Autodesk Fusion 360 part; units mm, degrees
sketch "Sketch1" plane through (0, 0, 0) normal (0, 0, 1) x (1, 0, 0)
  arc A0 (0.1047, -30.3528) -> (-0.0415, 30.353) centre (0, 0) ccw
  line L0 (-0.0415, 30.353) -> (-0.0415, 62.103)
  line L1 (0.1047, -30.3528) -> (0.1047, -62.1028)
  line L2 (-0.0415, 62.103) -> (57.1085, 62.103)
  line L3 (0.1047, -62.1028) -> (57.2547, -62.1028)
  line L4 (57.1085, 62.103) -> (57.2547, -62.1028)
  dimension "d1" = 60.706
  dimension "d10" = 31.75
  dimension "d12" = 57.15
extrude "Extrude1" add sketch "Sketch1" along normal mid plane 127
sketch "Sketch4" plane through (57.1815, 0.0673, 0) normal (1, 0.0012, 0) x (-0.0012, 1, 0)
  line L0 (62.0357, -63.5) -> (62.0357, 63.5)
  line L1 (62.0357, 63.5) -> (-62.1702, 63.5)
  line L2 (-62.1702, 63.5) -> (-62.1702, -63.5)
  line L3 (-62.1702, -63.5) -> (62.0357, -63.5)
  line L4 (57.15, -57.15) -> (-57.15, -57.15)
  line L5 (-57.15, -57.15) -> (-57.15, 57.15)
  line L6 (-57.15, 57.15) -> (-2.54, 57.15)
  line L7 (57.15, 6.35) -> (57.15, -57.15)
  line L8 (57.15, -57.15) -> (-57.15, 57.15) construction
  line L9 (-57.15, -57.15) -> (57.15, 57.15) construction
  line L10 (-2.54, 57.15) -> (-2.54, 6.35)
  line L11 (-2.54, 6.35) -> (57.15, 6.35)
  dimension "d21" = 114.3
  dimension "d22" = 114.3
  dimension "d35" = 59.69
  dimension "d36" = 50.8
extrude "Extrude3" cut sketch "Sketch4" against normal blind 25.4 contours L4 L5 L6 L7 L10 L11
sketch "Sketch6" plane through (57.1815, 0.0673, 0) normal (1, 0.0012, 0) x (-0.0012, 1, 0)
  line L0 (-57.15, 57.15) -> (-2.54, 57.15)
  line L1 (-2.54, 57.15) -> (-2.54, 6.35)
  line L2 (-2.54, 6.35) -> (57.15, 6.35)
  line L3 (57.15, 6.35) -> (57.15, -57.15)
  line L4 (57.15, -57.15) -> (-57.15, -57.15)
  line L5 (-57.15, -57.15) -> (-57.15, 57.15)
  line L6 (62.0357, -63.5) -> (62.0357, 63.5)
  line L7 (62.0357, 63.5) -> (-62.1702, 63.5)
  line L8 (-62.1702, 63.5) -> (-62.1702, -63.5)
  line L9 (-62.1702, -63.5) -> (62.0357, -63.5)
  line L10 (1.27, 57.15) -> (57.15, 57.15)
  line L11 (57.15, 57.15) -> (57.15, 8.89)
  line L12 (57.15, 8.89) -> (1.27, 8.89)
  line L13 (1.27, 8.89) -> (1.27, 57.15)
  dimension "d37" = 55.88
  dimension "d38" = 48.26
extrude "Extrude5" cut sketch "Sketch6" against normal blind 25.4 contours L10 L11 L12 L13
sketch "Sketch8" plane through (0, 0, 63.5) normal (0, 0, 1) x (-1, 0, 0)
  line L0 (-0.1047, 30.3528) -> (-0.1047, 62.1028)
  line L1 (-0.1047, 62.1028) -> (-57.2547, 62.1028)
  line L2 (-57.2547, 62.1028) -> (-57.1085, -62.103)
  line L3 (-57.1085, -62.103) -> (0.0415, -62.103)
  line L4 (0.0415, -62.103) -> (0.0415, -30.353)
  arc A0 (-0.1047, 30.3528) -> (0.0415, -30.353) centre (0, 0) ccw
  circle A1 centre (-49.9987, -11.1079) radius 0.8001
  circle A2 centre (-49.9987, -15.6799) radius 0.8001
  line L5 (-57.18, -1.3373) -> (-31.7801, -1.3074)
  dimension "d45" = 1.6002
  dimension "d46" = 4.572
  dimension "d47" = 9.779
extrude "Extrude6" cut sketch "Sketch8" against normal up to surface (6.35 mm away) contours A1 | A2
sketch "Sketch9" plane through (0.003, -2.54, 0) normal (0.0012, -1, 0) x (1, 0.0012, 0)
  line L0 (57.1816, 6.35) -> (57.1816, 57.15)
  line L1 (57.1816, 57.15) -> (31.7816, 57.15)
  line L2 (31.7816, 57.15) -> (31.7816, 6.35)
  line L3 (31.7816, 6.35) -> (57.1816, 6.35)
  line L4 (50.8316, 44.45) -> (38.1316, 44.45)
  line L5 (38.1316, 44.45) -> (38.1316, 19.05)
  line L6 (38.1316, 19.05) -> (50.8316, 19.05)
  line L7 (50.8316, 19.05) -> (50.8316, 44.45)
  dimension "d50" = 12.7
  dimension "d51" = 25.4
  dimension "d52" = 12.7
  dimension "d54" = 6.35
extrude "Extrude7" cut sketch "Sketch9" against normal up to surface (3.81 mm away) contours L4 L5 L6 L7
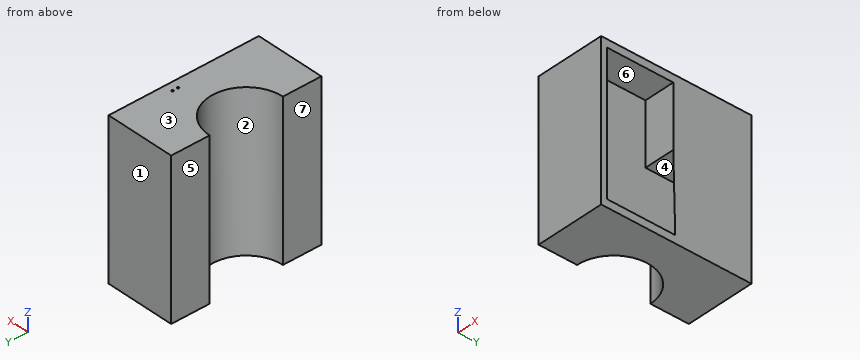
Part model, mm, in its own coordinate system. Face numbers are marked on the shaded views. A direction names the side the tool comes from. Coordinates: 2 decimals unless noted, no trailing zeros. Order: outer loops, then holes, each group sorted by start corner. A loop starts at its lowest first (then second) coordinate and runs counter-clockwise, first axis right, second up.
(1) Pull direction Y, two halves, no side cores. Call the marked faces 1, 2, 3 and 4: pulls with the +Y half, pulls with the -Y half, needs draft (parallel to the pull), parting line crosses it, or undercut.
Check sheet entries:
face 1: pulls with the +Y half
face 2: undercut
face 3: needs draft
face 4: undercut
(2) Slice it at D-D, the plane z = -5.5. Write the cut outline in (x, y), and give its area (3 significant figures).
Check sheet entries:
outline: (-0.04, 30.35) arc R30.35 cw to (0.1, -30.35) - (0.1, -62.1) - (57.25, -62.1) - (57.25, -57.08) - (31.85, -57.11) - (31.71, 57.19) - (57.11, 57.22) - (57.18, -0.84) - (57.11, 62.1) - (-0.04, 62.1) - close
area: 2,750 mm2
(3) Slice it at A-A, the plane x = 28.5. Write the cut outline in (y, z), and give its area (3 significant figures).
Check sheet entries:
outline: (-62.1, -63.5) - (-10.44, -63.5) - (-10.44, 63.5) - (-62.1, 63.5) - close; (10.44, -63.5) - (62.1, -63.5) - (62.1, 63.5) - (10.44, 63.5) - close
area: 13,100 mm2
(4) Slice it at C-C, the plane x = 41. Write the cut outline in (y, z).
Check sheet entries:
outline: (-62.1, -63.5) - (62.1, -63.5) - (62.1, 63.5) - (-62.1, 63.5) - close; hole (-57.1, -57.15) - (57.2, -57.15) - (57.2, 6.35) - (-2.49, 6.35) - (-2.49, 57.15) - (-57.1, 57.15) - close; hole (-2.49, 19.05) - (1.32, 19.05) - (1.32, 8.89) - (57.2, 8.89) - (57.2, 57.15) - (1.32, 57.15) - (1.32, 44.45) - (-2.49, 44.45) - close
(5) Probe L1, parallel to Y at x = 54.5, z = 55.5; L2, parallel to Z at x = 53.5, y = 39; L3, parallel to Z at x = 43.5, y = -3. List the from-to ranges inside material, lowest first.
Check sheet entries:
L1: y = -62.1 to -57.09, -2.48 to 1.33, 57.21 to 62.1
L2: z = -63.5 to -57.15, 6.35 to 8.89, 57.15 to 63.5
L3: z = -63.5 to -57.15, 57.15 to 63.5
(6) Slice it at B-B, the plane z = 54.5. Write the cut outline in (x, y).
Check sheet entries:
outline: (-0.04, 30.35) arc R30.35 cw to (0.1, -30.35) - (0.1, -62.1) - (57.25, -62.1) - (57.25, -57.08) - (31.85, -57.11) - (31.78, -2.5) - (57.18, -2.47) - (57.11, 62.1) - (-0.04, 62.1) - close; hole (31.71, 57.19) - (31.78, 1.31) - (57.18, 1.34) - (57.11, 57.22) - close
(7) Tool access for the marked faces 5, 6 and 7: list every direction of +Z, -Z, +X, -X, +Y, -Y with a clear straight run to the whole face (end or side of a thin tool).
Check sheet entries:
face 5: +Z, -Z, -X, +Y, -Y
face 6: +X
face 7: +Z, -Z, -X, -Y
(8) Pin check, flat tips, straight feed: pin 1 Ø6 at (y, z) = (-6.5, 36) entering from -X; pin 2 Ø4 at (y, z) = (-22.5, -14) entering from +X; pin 3 Ø2 at (y, z) = (41.5, -43.5) entering from +X. Stop position of each tip, or through.
Check sheet entries:
pin 1: stops at x = 28.83
pin 2: stops at x = 31.81
pin 3: stops at x = 57.13
